Verification items for the finished model (mm, model axes). Face numbers are marked on the shaded views. A direction names the side the tool comes from. Round coordinates to 2 decimals unless told otherwise and drop trailing zeros. Loops run counter-clockwise (first coordinate to the right, second up) from the corner with the lowest first, then second, coordinate; pieces in that order, holes last. Notation, with made-up numbers: M 81.25,76 L 95.25,76 A30 ccw 95.25,102 Z; hole C 22,76.25 d7. An arc over 180 degrees is marked long. Write item = value, one per line. Start each with the question number.
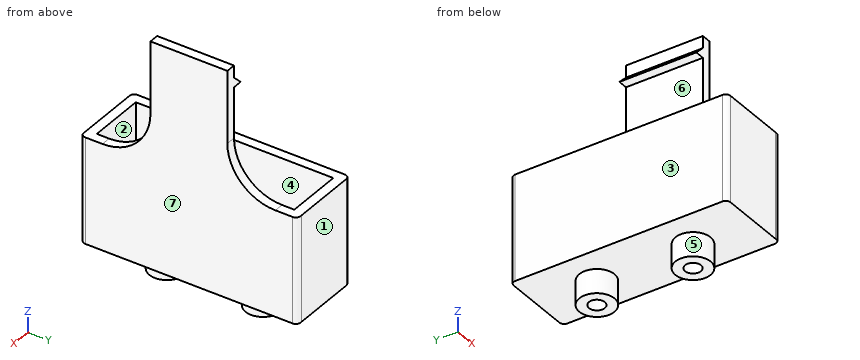
from build123d import *

# Parameters (mm, degrees)
SKETCH1_R             = 3.66
SKETCH1_R_2           = 1.65
BOSS_EXTRUDE1_DEPTH   = 5
BOSS_EXTRUDE1_2_DEPTH = 5
SKETCH2_R             = 1.65
BOSS_EXTRUDE2_DEPTH   = 22
SKETCH3_W             = 11.8
SKETCH3_H             = 41.1
CUT_EXTRUDE1_DEPTH    = 20
SKETCH4_W             = 2.01
SKETCH4_H             = 16
BOSS_EXTRUDE3_DEPTH   = 25
FILLET1_R             = 10
BOSS_EXTRUDE4_DEPTH   = 16


with BuildPart() as part:
    # Sketch1 → Boss-Extrude1 (new body)
    with BuildSketch(Plane.XY):
        with Locations((0, -9.999161717)):
            Circle(SKETCH1_R)
        with Locations((0, -9.999161717)):
            Circle(SKETCH1_R_2, mode=Mode.SUBTRACT)
    extrude(amount=BOSS_EXTRUDE1_DEPTH)



with BuildPart() as body_2:
    # Sketch1 → Boss-Extrude1 2 (new body)
    with BuildSketch(Plane.XY):
        with Locations((0, 9.999161717)):
            Circle(SKETCH1_R)
        with Locations((0, 9.999161717)):
            Circle(SKETCH1_R_2, mode=Mode.SUBTRACT)
    extrude(amount=BOSS_EXTRUDE1_2_DEPTH)


with BuildPart() as part_1:
    add(part.part)

    add(body_2.part)  # Boss-Extrude2 merges body 2
    # Sketch2 → Boss-Extrude2 (add)
    with BuildSketch(Plane.XY.offset(5)):
        with BuildLine():
            Line((-6.91, 22.56), (6.71, 22.56))
            ThreePointArc((6.71, 22.56), (7.550387634, 22.348468599), (7.91, 21.560004361))
            Line((7.91, 21.560004361), (7.91, -21.560004361))
            ThreePointArc((7.91, -21.560004361), (7.550387634, -22.348468599), (6.71, -22.56))
            Line((6.71, -22.56), (-6.91, -22.56))
            ThreePointArc((-6.91, -22.56), (-7.617106781, -22.267106781), (-7.91, -21.56))
            Line((-7.91, -21.56), (-7.91, 21.56))
            ThreePointArc((-7.91, 21.56), (-7.617106781, 22.267106781), (-6.91, 22.56))
        make_face()
        with Locations((0, 9.999161717)):
            Circle(SKETCH2_R, mode=Mode.SUBTRACT)
        with Locations((0, -9.999161717)):
            Circle(SKETCH2_R, mode=Mode.SUBTRACT)
    extrude(amount=BOSS_EXTRUDE2_DEPTH)

    # Sketch3 → Cut-Extrude1 (cut)
    with BuildSketch(Plane.XY.offset(27)):
        Rectangle(SKETCH3_W, SKETCH3_H)
    extrude(amount=-CUT_EXTRUDE1_DEPTH, mode=Mode.SUBTRACT)

    # Sketch4 → Boss-Extrude3 (add)
    with BuildSketch(Plane.XY.offset(27)):
        with Locations((6.905, 0)):
            Rectangle(SKETCH4_W, SKETCH4_H)
    extrude(amount=BOSS_EXTRUDE3_DEPTH)

    # Fillet1
    fillet1_edges = [part_1.edges().sort_by_distance(p)[0] for p in [
        (6.905, -8, 27),
        (6.905, 8, 27),
    ]]
    fillet(fillet1_edges, radius=FILLET1_R)

    # Sketch5 → Boss-Extrude4 (add)
    with BuildSketch(Plane.XZ.offset(8)):
        Polygon((5.9, 47.5), (3.9, 47.5), (5.9, 49.5), align=None)
    extrude(amount=-BOSS_EXTRUDE4_DEPTH)


solid = part_1.part
1. Section check A-A, the plane x = 0. Enter the section's corners in (y, z).
2. Thickness scan on line 1 (Y direction, x = 0, z = 3.25); line 2 (Y direction, x = -2.75, z = 10); line 3 (X direction, y = -9, z = 22.5). Record the ranges inside material, lowest first.
3. Section check B-B, the plane z = 20. Enter the section's corners in (x, y), and give its area (3 significant figures).
4. Section check D-D, the plane y = 4. Enter the section's corners in (x, z), and give its area (3 significant figures).
5. Section check C-C, the plane x = -4.75. Enter the section's corners in (y, z).
6. Tool access check on the marked faces 4, 5, 6 and 7. Record the directions out of +Z, -Z, +X, -X, +Y, -Y that give a thin tool (end or side, any length) a straight path to the whole face; none if there is none.
7. Gauge pin test, flat ends, axial feed: P1, Ø6, axis at x = -5, y = 0.5, coming from the -Z side; P2, Ø6, axis at x = 6, y = -16, coming from the +Z side; P3, Ø4, axis at x = -3, z = 11.5, coming from the -Y side; P4, Ø2.5, axis at x = 0, y = 10, coming from the -Z side. Record the tip position at first contact, or that the pin passes through.
8. Mould release check, pull along X, two halves, no side actions. Record for the marked faces 1, 2 and 3: pulls with the +X half, pulls with the -X half, needs draft (parallel to the pull), parting line crosses it, or undercut.
Computed values:
q1.outline = M -22.56,5 L -13.66,5 L -13.66,0 L -11.65,0 L -11.65,7 L -20.55,7 L -20.55,27 L -22.56,27 Z; M -8.35,0 L -6.34,0 L -6.34,5 L 6.34,5 L 6.34,0 L 8.35,0 L 8.35,7 L -8.35,7 Z; M 11.65,0 L 13.66,0 L 13.66,5 L 22.56,5 L 22.56,27 L 20.55,27 L 20.55,7 L 11.65,7 Z
q2.line_1 = -13.66 to -11.65, -8.35 to -6.34, 6.34 to 8.35, 11.65 to 13.66
q2.line_2 = -22.56 to -20.55, 20.55 to 22.56
q2.line_3 = -7.91 to -5.9, 5.9 to 7.91
q3.outline = M -7.91,-21.56 A1 ccw -6.91,-22.56 L 6.71,-22.56 A1 ccw 7.91,-21.56 L 7.91,21.56 A1 ccw 6.71,22.56 L -6.91,22.56 A1 ccw -7.91,21.56 Z; hole M -5.9,-20.55 L 5.9,-20.55 L 5.9,20.55 L -5.9,20.55 Z
q3.area = 228 mm2
q4.outline = M -7.91,5 L 7.91,5 L 7.91,52 L 5.9,52 L 5.9,49.5 L 3.9,47.5 L 5.9,47.5 L 5.9,7 L -5.9,7 L -5.9,27 L -7.91,27 Z
q4.area = 164 mm2
q5.outline = M -22.56,5 L 22.56,5 L 22.56,27 L 20.55,27 L 20.55,7 L -20.55,7 L -20.55,27 L -22.56,27 Z
q6.face_4 = +Z
q6.face_5 = -Z
q6.face_6 = none
q6.face_7 = +Z, -Z, +X, +Y, -Y
q7.P1 = 5
q7.P2 = 28.34
q7.P3 = -22.56
q7.P4 = through
q8.face_1 = needs draft
q8.face_2 = undercut
q8.face_3 = pulls with the -X half
